```python
from build123d import *

# Parameters (mm, degrees)
SKETCH_4_W          = 26.5
SKETCH_4_H          = 26.5
SKETCH_4_W_2        = 20.5
SKETCH_4_H_2        = 20.5
EXTRUDE_1_DEPTH     = 50
EXTRUDE_2_DEPTH     = 50
EXTRUDE_3_DEPTH     = 17.5
SKETCH_4_2_W        = 20.5
SKETCH_4_2_H        = 20.5
CUT_EXTRUDE_1_DEPTH = 82.971372719
CUT_EXTRUDE_2_DEPTH = 82.971372719
SKETCH_7_R          = 1.5
CUT_EXTRUDE_3_DEPTH = 93.625217786
SKETCH_8_R          = 1.6
CUT_EXTRUDE_4_DEPTH = 76.350501248


with BuildPart() as part:
    # Sketch 4 → Extrude 1 (new body)
    with BuildSketch(Plane(origin=(0, 0, 0), x_dir=(1, 0, 0), z_dir=(0, 1, 0))):
        Rectangle(SKETCH_4_W, SKETCH_4_H)
        Rectangle(SKETCH_4_W_2, SKETCH_4_H_2, mode=Mode.SUBTRACT)
    extrude(amount=-EXTRUDE_1_DEPTH)

    # Sketch 5 → Extrude 2 (add)
    with BuildSketch(Plane(origin=(0, 0, 0), x_dir=(0.7254762501100117, 0.21764287503300356, -0.6529286250990104), z_dir=(0.6882472016116853, -0.22941573387056186, 0.6882472016116854))):
        Polygon((15.877292577, 9.951712437), (9.951712437, -15.877292577), (-15.877292577, -9.951712437), (-9.951712437, 15.877292577), align=None)
        Polygon((-7.698494526, 12.28243388), (12.28243388, 7.698494526), (7.698494526, -12.28243388), (-12.28243388, -7.698494526), align=None, mode=Mode.SUBTRACT)
    extrude(amount=-EXTRUDE_2_DEPTH)

    # Sketch 6 → Extrude 3 (add, symmetric)
    with BuildSketch(Plane(origin=(0, 0, 0), x_dir=(1, 0, 0), z_dir=(0, 1, 0))):
        Polygon((13.25, -13.25), (-21.75, -13.25), (-21.75, 3.011670299), (-3.011670299, 21.75), (13.25, 21.75), align=None)
    extrude(amount=EXTRUDE_3_DEPTH, both=True)

    # Sketch 4_2 → Cut-Extrude 1 (cut, through all)
    with BuildSketch(Plane(origin=(0, 0, 0), x_dir=(1, 0, 0), z_dir=(0, 1, 0))):
        Rectangle(SKETCH_4_2_W, SKETCH_4_2_H)
    extrude(amount=-CUT_EXTRUDE_1_DEPTH, mode=Mode.SUBTRACT)

    # Sketch 5_2 → Cut-Extrude 2 (cut, through all)
    with BuildSketch(Plane(origin=(0, 0, 0), x_dir=(0.7254762501100117, 0.21764287503300356, -0.6529286250990104), z_dir=(0.6882472016116853, -0.22941573387056186, 0.6882472016116854))):
        Polygon((12.28243388, 7.698494526), (7.698494526, -12.28243388), (-12.28243388, -7.698494526), (-7.698494526, 12.28243388), align=None)
    extrude(amount=-CUT_EXTRUDE_2_DEPTH, mode=Mode.SUBTRACT)

    # Sketch 7 → Cut-Extrude 3 (cut, through all)
    with BuildSketch(Plane(origin=(2.14943383, 12.89660298, 2.14943383), x_dir=(0.9867543820659302, -0.16001422411879954, -0.026669037353133265), z_dir=(0.1622214211307626, 0.9733285267845754, 0.1622214211307625))):
        with Locations(Location((-31.386862461, 32.246935744, 0), (0, 0, 178.451276833))):
            Circle(SKETCH_7_R)
        with Locations(Location((-20.924574974, 21.497957163, 0), (0, 0, 178.451276833))):
            Circle(SKETCH_7_R)
    extrude(amount=-CUT_EXTRUDE_3_DEPTH, mode=Mode.SUBTRACT)

    # Sketch 8 → Cut-Extrude 4 (cut, through all)
    with BuildSketch(Plane.ZY.offset(13.25)):
        with Locations((0, -22.5)):
            Circle(SKETCH_8_R)
        with Locations((0, -42.5)):
            Circle(SKETCH_8_R)
    extrude(amount=-CUT_EXTRUDE_4_DEPTH, mode=Mode.SUBTRACT)


solid = part.part
```
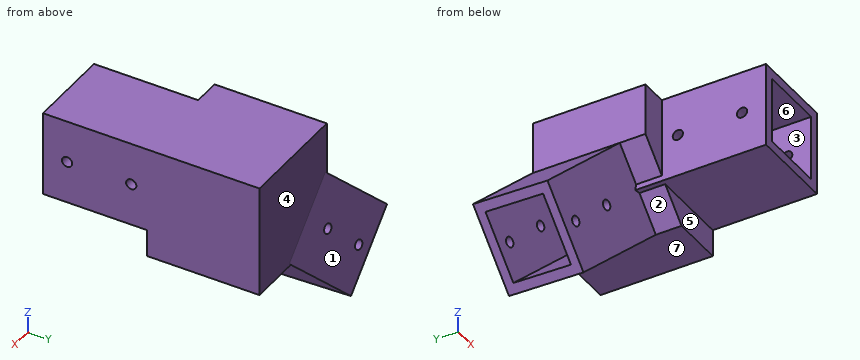
Input: part model. Units: mm. Frame: model coordinates. Face numbers are marked on the shaded views. A direction names the side the tool comes from. Round coordinates to 2 decimals unless told otherwise and drop trailing zeros. Write each loop counter-clockwise with the first axis right and the second up, starting at its lowest first coordinate (ties: lowest second). Pieces come first, ordered by that corner, then holes. Notation, with made-up numbers: (-23, -6.5) - (-2, -6.5) arc R17 ccw to (-2, 3.5) - close; hole circle Ø9 at (63, -19). An arc over 180 degrees is marked (long way). Write item = value, one per line.
(1) Section query C-C on z = 0. State how many separate pieces and enclosed holes the cut face has, then the cut area to 3 significant figures.
Geometry check:
separate_pieces = 5
enclosed_holes = 0
area = 799 mm^2
(2) Section query D-D on z = 6. Output: boundary loops of the cut face in (x, y).
Geometry check:
outline = (-21.75, -17.5) - (-13.25, -17.5) - (-13.25, -50) - (-10.25, -50) - (-10.25, 0) - (-8.5, 0) - (-8.5, 10.95) - (-2.67, 9.98) - (-6, 0) - (10.25, 0) - (10.25, -50) - (13.25, -50) - (13.25, 17.5) - (-21.75, 17.5) - close
(3) Contact query for flat-ended pins moving along their axis: pin 1 Ø5 at (y, z) = (1.5, 3) entering from -X; pin 2 Ø2 at (x, z) = (-11.5, -0.5) entering from +Y; pin 3 Ø5 at (x, z) = (-1.5, -4) entering from -Y; pin 4 Ø8 at (x, z) = (-29, 3.5) entering from -Y. Output: stop coordinate, or through.
Geometry check:
pin_1 = -21.75
pin_2 = 17.5
pin_3 = 10.86
pin_4 = through
(4) Access query for the marked faces 5, 6 and 7. Directions: +Z, -Z, +X, -X, +Y, -Y. A direction counts if a zero-diameter tool reaches every point of the face in a straight line with its end or side. Return the directions, or none.
Geometry check:
face_5 = -Z, +X, -X, -Y
face_6 = -Y
face_7 = -Z, +X, +Y, -Y
(5) Section query B-B on y = -42.5. Output: boundary loops of the cut face in (x, z), then the cut area to 3 significant figures.
Geometry check:
outline = (-13.25, -13.25) - (13.25, -13.25) - (13.25, -1.6) - (10.25, -1.6) - (10.25, -10.25) - (-10.25, -10.25) - (-10.25, -1.6) - (-13.25, -1.6) - close; (-13.25, 1.6) - (-10.25, 1.6) - (-10.25, 10.25) - (10.25, 10.25) - (10.25, 1.6) - (13.25, 1.6) - (13.25, 13.25) - (-13.25, 13.25) - close
area = 263 mm^2
(6) Pull-direction query (Z, two-part tool) for the marked faces 1, 2, 3 and 4; classes: +Z half, -Z half, draft (parallel to the pull), parting line (faces both ways), or undercut.
Geometry check:
face_1 = +Z half
face_2 = -Z half
face_3 = undercut
face_4 = draft
(7) Section query A-A on y = -34.5. Output: boundary loops of the cut face in (x, z), then the cut area to 3 significant figures.
Geometry check:
outline = (-13.25, -13.25) - (13.25, -13.25) - (13.25, 13.25) - (-13.25, 13.25) - close; hole (-10.25, -10.25) - (10.25, -10.25) - (10.25, 10.25) - (-10.25, 10.25) - close
area = 282 mm^2
(8) Material intervals for probe 1 along Y at (x, z) = (12, 0); probe 2 along Z at (x, y) = (7, -20.5); probe 3 along Y at (x, z) = (-11.1, 0), sorted ascending.
Geometry check:
probe_1 = -50 to -44.1, -40.9 to -24.1, -20.9 to 17.5
probe_2 = -13.25 to -10.25, 10.25 to 13.25
probe_3 = -50 to -44.1, -40.9 to -24.1, -20.9 to -8.68, 12.38 to 17.5
